Build history of the part. All positions in model axes, mm. Face numbers are marked on the shaded views. A direction names the side the tool comes from. Give positions to 0.01 mm unless a question says otherwise; leave off trailing zeros. Return JSON: item names as keys, results as strings. Group by question number.
1) Drop flat-ended pins along their axis: pin 1 (1 mm diameter, centred on x = 13.5, z = 8.5, fed in from -Y); pin 2 (5 mm diameter, centred on x = -0.5, z = 24.5, fed in from -Y); pin 3 (4 mm diameter, centred on y = 1.5, z = 18.5, fed in from +X); pin 4 (10 mm diameter, centred on x = 3.5, y = -15, fed in from -Z). Give the stop position or say it passes through.
2) Drill centre lines: probe 1 along X at (y, z) = (24, 7); probe 2 along Y at (x, z) = (19.5, 6.5); probe 3 along X at (y, z) = (20, 4). Where is each one in solid material? Low to high. Write a range as from..to.
3) 3-axis set-ups, long thin cutter, end or side, ignore diameter. For the marked faces 1, 2 and 3: which of +Z, -Z, +X, -X, +Y, -Y reach the whole face in a straight line?
4) Mould opens along X. For the marked faces 4, 5 and 6 say: released by +X, released by -X, zero draft, split by the parting line, or undercut.
```python
from build123d import *

# Parameters (mm, degrees)
F3_W           = 110.9925583005
F3_H           = 44.4556474686
F4_DEPTH       = 40
F4_DEPTH_BACK  = 40
F7_DEPTH       = 60
F7_DEPTH_BACK  = 25
F12_DEPTH      = 60
F12_DEPTH_BACK = 60
F16_DEPTH      = 60
F16_DEPTH_BACK = 60


with BuildPart() as f2:
    # F0 (on Top) → F2 (revolve)
    with BuildSketch(Plane.XY):
        with BuildLine():
            Line((0, 35), (0, -35))
            ThreePointArc((0, -35), (35, 0), (0, 35))
        make_face()
    revolve(axis=Axis((0, 0, 0), (0, -1, 0)))

    # F3 (on Front) → F4 (cut, two sides)
    with BuildSketch(Plane.XZ) as f4_sk:
        with Locations((0.8793435991, -22.2278237343)):
            Rectangle(F3_W, F3_H)
    extrude(amount=-F4_DEPTH, mode=Mode.SUBTRACT)
    extrude(f4_sk.sketch, amount=F4_DEPTH_BACK, mode=Mode.SUBTRACT)

    # F6 (on line) → F7 (cut, two sides)
    with BuildSketch(Plane(origin=(0, 0, 0), x_dir=(0.8660254038, 0, 0.5), z_dir=(0.5, 0, -0.8660254038))) as f7_sk:
        with BuildLine():
            Line((12.7, -40.8236384392), (12.7, -17.7161854768))
            ThreePointArc((12.7, -17.7161854768), (0, -5.0161854768), (-12.7, -17.7161854768))
            Line((-12.7, -17.7161854768), (-12.7, -40.8236384392))
            Line((-12.7, -40.8236384392), (12.7, -40.8236384392))
        make_face()
    extrude(amount=-F7_DEPTH, mode=Mode.SUBTRACT)
    extrude(f7_sk.sketch, amount=F7_DEPTH_BACK, mode=Mode.SUBTRACT)

    # F11 (on line) → F12 (cut, two sides)
    with BuildSketch(Plane(origin=(0, 0, 0), x_dir=(0.9682458366, 0.1118033989, -0.2236067977), z_dir=(-0.25, 0.4330127019, -0.8660254038))) as f12_sk:
        with BuildLine():
            Line((-36.9845643478, 4.2932505168), (-21.3320885053, -3.5329874044))
            ThreePointArc((-21.3320885053, -3.5329874044), (-4.2932505168, 2.1466252584), (-9.9728631796, 19.1854632469))
            Line((-9.9728631796, 19.1854632469), (-25.6253390221, 27.0117011682))
            Line((-25.6253390221, 27.0117011682), (-36.9845643478, 4.2932505168))
        make_face()
    extrude(amount=-F12_DEPTH, mode=Mode.SUBTRACT)
    extrude(f12_sk.sketch, amount=F12_DEPTH_BACK, mode=Mode.SUBTRACT)

    # F15 (on line) → F16 (cut, two sides)
    with BuildSketch(Plane(origin=(0, 0, 0), x_dir=(0.9682458366, -0.1118033989, -0.2236067977), z_dir=(-0.25, -0.4330127019, -0.8660254038))) as f16_sk:
        with BuildLine():
            Line((25.6253390221, 27.0117011682), (9.9728631796, 19.1854632469))
            ThreePointArc((9.9728631796, 19.1854632469), (4.2932505168, 2.1466252584), (21.3320885053, -3.5329874044))
            Line((21.3320885053, -3.5329874044), (36.9845643478, 4.2932505168))
            Line((36.9845643478, 4.2932505168), (25.6253390221, 27.0117011682))
        make_face()
    extrude(amount=-F16_DEPTH, mode=Mode.SUBTRACT)
    extrude(f16_sk.sketch, amount=F16_DEPTH_BACK, mode=Mode.SUBTRACT)


solid = f2.part
```
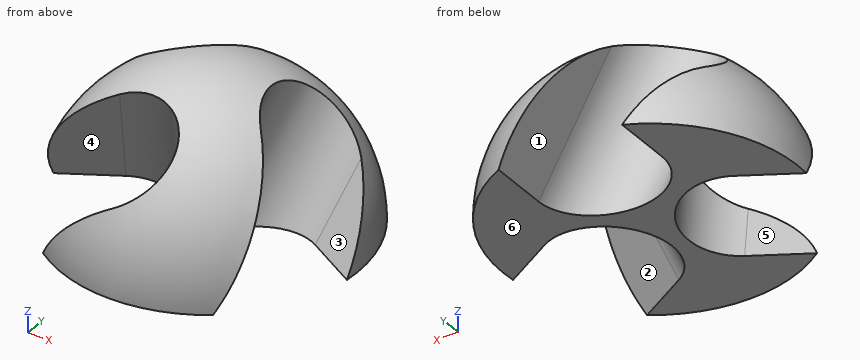
Results:
{
 "1": {"pin 1": "y = -31.4", "pin 2": "y = -13.24", "pin 3": "x = 8.09", "pin 4": "z = 0"},
 "2": {"probe 1": "-24.49..-18.71, 10.62..24.49", "probe 2": "-28.33..-23.86, 8.67..28.33", "probe 3": "-28.44..-16.97, 12.36..28.44"},
 "3": {"face 1": "-Z, +Y", "face 2": "-Z, +X", "face 3": "+Z, -Y"},
 "4": {"face 4": "undercut", "face 5": "released by -X", "face 6": "zero draft"}
}
